Design review of the part built by this model. Coordinates are the model's own, in mm. A direction names the side the tool comes from. Round coordinates to 2 decimals unless told otherwise and drop trailing zeros. Loops run counter-clockwise (first coordinate to the right, second up) from the corner with the lowest first, then second, coordinate; pieces in that order, holes last. Notation, with made-up numbers: M 1,5 L 34,5 A15 cw 34,20 Z; hole C 47,-16 d2. An arc over 180 degrees is marked long. One line per item, written item: value. Start each with the question number.
Item 1: Mouldability with a two-part tool opening along Z and no side actions: class faces 4 (the flat face through (-44, 11, -23.185)), 5 (the flat face through (-47, 1.61, -6)), 6 (the cylindrical face through (-46.886, 15.302, 9.839)), 7 (the cylindrical face through (-47.422, 11.313, 10.363)) as released by +Z, released by -Z, zero draft, split by the parting line, or undercut.
Item 2: We need section C-C (z = -5). Write out the cut boundary in (x, y) (3 decimals), then the cut area to 3 significant figures.
Item 3: We need section A-A (y = 9.25). Write out the cut boundary in (x, z) (3 decimals).
Item 4: Clearance check with flat-ended pins moving along their axes: pin 1 (2.5 mm diameter, centred on y = 5.5, z = -7.5, fed in from +X); pin 2 (5.5 mm diameter, centred on y = 16, z = -8, fed in from +X) (3 decimals); pin 3 (2 mm diameter, centred on x = -44.5, z = -11.5, fed in from +Y). State where each tip first meets the part, or that it passes through.
Item 5: For faces 1 (the flat face through (-48.135, 11, -6)), 2 (the flat face through (-46.47, 6, -6)), 3 (the flat face through (-44, 15, 10.365)), list the 3-axis set-ups (+Z, -Z, +X, -X, +Y, -Y) from which the entire face can be reached by the end or side of a thin tool; tool diameter is ignored.
Item 6: We need section D-D (y = 14). Write out the cut boundary in (x, z) (3 decimals).
Item 7: We need section B-B (x = -44.4). Write out the cut boundary in (y, z) (3 decimals).
Item 8: For line 1 along Z through (x, y) = (-44.05, 15) (3 decimals); line 2 along Z through (x, y) = (-44.2, 6) (3 decimals); line 3 along Y through (x, z) = (-46.1, -19.5), list the stretches that pass through material, from the lowest coordinate up.
from build123d import *

# Parameters (mm, degrees)
SKETCH2_W           = 5.08
SKETCH2_H           = 34.3
BOSS_EXTRUDE1_DEPTH = 19.1389
FILLET1_R           = 2.5
SKETCH3_W           = 3.415
SKETCH3_H           = 24.61
CUT_EXTRUDE1_DEPTH  = 55.558231654
CUT_EXTRUDE2_DEPTH  = 11.0489


with BuildPart() as part:
    # Sketch2 → Boss-Extrude1 (new body)
    with BuildSketch(Plane(origin=(0, 1.61, 0), x_dir=(1, 0, 0), z_dir=(0, 1, 0))):
        with Locations((-45.595, 6.035)):
            Rectangle(SKETCH2_W, SKETCH2_H)
    extrude(amount=BOSS_EXTRUDE1_DEPTH)

    # Fillet1
    fillet1_edges = [part.edges().sort_by_distance(p)[0] for p in [
        (-48.135, 11.17945, -23.185),
        (-48.135, 11.17945, 11.115),
    ]]
    fillet(fillet1_edges, radius=FILLET1_R)

    # Sketch3 → Cut-Extrude1 (cut, through all)
    with BuildSketch(Plane(origin=(0, 9.7, 0), x_dir=(-1, 0, 0), z_dir=(0, -1, 0))):
        with Locations((44.7625, 6.035)):
            Rectangle(SKETCH3_W, SKETCH3_H)
    extrude(amount=CUT_EXTRUDE1_DEPTH, mode=Mode.SUBTRACT)

    # Sketch4 → Cut-Extrude2 (cut)
    with BuildSketch(Plane(origin=(0, 20.7489, 0), x_dir=(1, 0, 0), z_dir=(0, 1, 0))):
        with BuildLine():
            Line((-43.055, -10.365), (-43.055, 22.435))
            Line((-43.055, 22.435), (-45.635, 22.435))
            ThreePointArc((-45.635, 22.435), (-46.872436867, 21.922436867), (-47.385, 20.685))
            Line((-47.385, 20.685), (-47.385, -8.615))
            ThreePointArc((-47.385, -8.615), (-46.872436867, -9.852436867), (-45.635, -10.365))
            Line((-45.635, -10.365), (-43.055, -10.365))
        make_face()
    extrude(amount=-CUT_EXTRUDE2_DEPTH, mode=Mode.SUBTRACT)


solid = part.part
A:
1. face 4: released by -Z
1. face 5: zero draft
1. face 6: undercut
1. face 7: released by +Z
2. outline: M -48.135,1.61 L -46.47,1.61 L -46.47,9.7 L -47.385,9.7 L -47.385,20.749 L -48.135,20.749 Z
2. area: 21.8 mm2
3. outline: M -48.135,-20.685 A2.5 ccw -45.635,-23.185 L -43.055,-23.185 L -43.055,-18.34 L -46.47,-18.34 L -46.47,6.27 L -43.055,6.27 L -43.055,11.115 L -45.635,11.115 A2.5 ccw -48.135,8.615 Z
4. pin 1: x = -46.47
4. pin 2: x = -47.385
4. pin 3: through
5. face 1: +Z, -Z, -X, +Y, -Y
5. face 2: +X, +Y, -Y
5. face 3: +X, +Y
6. outline: M -48.135,-20.685 A2.5 ccw -45.635,-23.185 L -43.055,-23.185 L -43.055,-22.435 L -45.635,-22.435 A1.75 cw -47.385,-20.685 L -47.385,8.615 A1.75 cw -45.635,10.365 L -43.055,10.365 L -43.055,11.115 L -45.635,11.115 A2.5 ccw -48.135,8.615 Z
7. outline: M 1.61,-23.185 L 20.749,-23.185 L 20.749,-22.435 L 9.7,-22.435 L 9.7,-18.34 L 1.61,-18.34 Z; M 1.61,6.27 L 9.7,6.27 L 9.7,10.365 L 20.749,10.365 L 20.749,11.115 L 1.61,11.115 Z
8. line 1: -23.185 to -22.435, 10.365 to 11.115
8. line 2: -23.185 to -18.34, 6.27 to 11.115
8. line 3: 1.61 to 9.7
